from build123d import *

# Parameters (mm, degrees)
F1_DEPTH = 55
F2_R     = 15.559852
F3_R     = 5


with BuildPart() as f1:
    # F0 (on Front) → F1 (new body)
    with BuildSketch(Plane.XZ):
        Polygon((-80, 0), (0, 0), (0, 80), align=None)
    extrude(amount=F1_DEPTH)

    # F2
    f2_edges = [f1.edges().sort_by_distance(p)[0] for p in [
        (0, -27.5, 80),
    ]]
    fillet(f2_edges, radius=F2_R)

    # F3
    f3_edges = [f1.edges().sort_by_distance(p)[0] for p in [
        (0, -55, 21.217598),
        (0, 0, 21.217598),
        (0, -27.5, 0),
    ]]
    fillet(f3_edges, radius=F3_R)


solid = f1.part
Check sheet for the modelled part. Datum: model origin and axes. Units: mm. Round coordinates to 2 decimals unless told otherwise and drop trailing zeros. Order: outer loops, then holes, each group sorted by start corner. A loop starts at its lowest first (then second) coordinate and runs counter-clockwise, first axis right, second up.
Q1. Depth check by flat-ended pin: P1, Ø3, axis at y = -39, z = 47, coming from the +X side; P2, Ø1.5, axis at y = -40, z = 49.5, coming from the +X side; P3, Ø2, axis at x = -35, y = -19, coming from the +Z side. Enter the tip coordinate at first touch or a pass-through.
Filled sheet:
P1: stops at x = -0.3
P2: stops at x = -1.34
P3: stops at z = 46
Q2. Scan lines: L1, parallel to Z at x = -15, y = -5; L2, parallel to X at y = -48, z = 33; L3, parallel to X at y = -44, z = 7. Record each from-to range of solid material in increasing order.
Filled sheet:
L1: z = 0 to 57.98
L2: x = -47 to 0
L3: x = -73 to 0
Q3. Cross-section at A-A, the plane y = -17. Enter the section's corners in (x, z), plus the area to 3 significant figures.
Filled sheet:
outline: (-80, 0) - (-5, 0) arc R5 ccw to (0, 5) - (0, 42.44) arc R15.56 ccw to (-26.56, 53.44) - close
area: 2,900 mm2
